The listing builds one solid part. Answer for the finished solid, in the listing's coordinates (mm). Face numbers are marked on the shaded views. A direction names the side the tool comes from. Coordinates: 2 decimals unless noted, no trailing zeros. Write each loop counter-clockwise with the first axis right and the second up, starting at its lowest first coordinate (ties: lowest second). Pieces come first, ordered by that corner, then holes. Notation, with made-up numbers: M -34,39 L -1,39 A24 ccw -1,58 Z; hole C -0.75,34 d1. An arc over 180 degrees is marked long. Put each result on its own line as item: value. Start each with the question number.
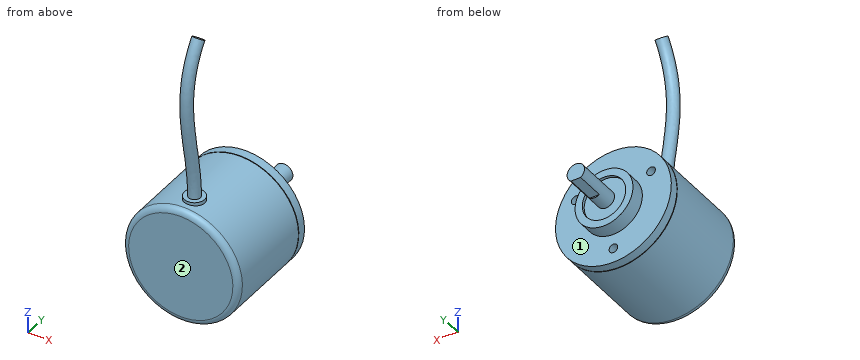
```python
from build123d import *

# Parameters (mm, degrees)
SKETCH1_R           = 20
BOSS_EXTRUDE1_DEPTH = 35
SKETCH3_R           = 10
BOSS_EXTRUDE3_DEPTH = 5
SKETCH4_R           = 7.5
CUT_EXTRUDE1_DEPTH  = 1
SKETCH5_R           = 3
BOSS_EXTRUDE4_DEPTH = 16
SKETCH6_W           = 5.83666228
SKETCH6_H           = 4.189609368
CUT_EXTRUDE2_DEPTH  = 10
SKETCH10_W          = 2.171108564
SKETCH10_H          = 0.2
SKETCH11_R          = 3.5
BOSS_EXTRUDE5_DEPTH = 21
SKETCH12_R          = 2
FILLET1_R           = 2
SKETCH24_R          = 1.5
CUT_EXTRUDE3_DEPTH  = 6


with BuildPart() as part:
    # Sketch1 → Boss-Extrude1 (new body)
    with BuildSketch(Plane(origin=(0, 0, 0), x_dir=(1, 0, 0), z_dir=(0, 1, 0))):
        with Locations(Location((0, 0, 0), (0, 0, 270))):
            Circle(SKETCH1_R)
    extrude(amount=BOSS_EXTRUDE1_DEPTH)

    # Sketch3 → Boss-Extrude3 (add)
    with BuildSketch(Plane(origin=(0, 35, 0), x_dir=(1, 0, 0), z_dir=(0, 1, 0))):
        with Locations(Location((0, 0, 0), (0, 0, 270))):
            Circle(SKETCH3_R)
    extrude(amount=BOSS_EXTRUDE3_DEPTH)

    # Sketch4 → Cut-Extrude1 (cut)
    with BuildSketch(Plane(origin=(0, 40, 0), x_dir=(1, 0, 0), z_dir=(0, 1, 0))):
        with Locations(Location((0, 0, 0), (0, 0, 270))):
            Circle(SKETCH4_R)
    extrude(amount=-CUT_EXTRUDE1_DEPTH, mode=Mode.SUBTRACT)

    # Sketch5 → Boss-Extrude4 (add)
    with BuildSketch(Plane(origin=(0, 39, 0), x_dir=(1, 0, 0), z_dir=(0, 1, 0))):
        with Locations(Location((0, 0, 0), (0, 0, 270))):
            Circle(SKETCH5_R)
    extrude(amount=BOSS_EXTRUDE4_DEPTH)

    # Sketch6 → Cut-Extrude2 (cut)
    with BuildSketch(Plane(origin=(0, 55, 0), x_dir=(1, 0, 0), z_dir=(0, 1, 0))):
        with Locations((0, 4.594804684)):
            Rectangle(SKETCH6_W, SKETCH6_H)
    extrude(amount=-CUT_EXTRUDE2_DEPTH, mode=Mode.SUBTRACT)

    # Sketch10 → Cut-Revolve1 (revolve, cut)
    with BuildSketch(Plane.XY, mode=Mode.PRIVATE) as cut_revolve1_sk:
        with Locations((20, 31.9)):
            Rectangle(SKETCH10_W, SKETCH10_H)
    revolve(cut_revolve1_sk.sketch.rotate(Axis((0, 0, 0), (0, 1, 0)), 123.557309762), axis=Axis((0, 0, 0), (0, 1, 0)), mode=Mode.SUBTRACT)

    # Sketch11 → Boss-Extrude5 (add)
    with BuildSketch(Plane.XY):
        with Locations(Location((0, 7.305759765, 0), (0, 0, 180))):
            Circle(SKETCH11_R)
    extrude(amount=BOSS_EXTRUDE5_DEPTH)

    # Sweep1: sweep along a path in Sketch13
    with BuildLine() as sweep1_path:  # in the path sketch's own coordinates; laid on its plane below (add() does not lay a ready-made edge on the line's plane)
        add(Edge.make_bspline(
            [(-21, 7.305759765), (-39.680829044, 7.305759765), (-58.658536918, -3.239081936), (-76.270922844, 9.376545434)],
            knots=[0, 0, 0, 0, 1, 1, 1, 1], degree=3))
    # Sketch12 → Sweep1 (sweep)
    with BuildSketch(Plane.XY.offset(21)):
        with Locations((0, 7.305759765)):
            Circle(SKETCH12_R)
    sweep(path=Plane(origin=(0, 0, 0), x_dir=(0, 0, -1), z_dir=(1, 0, 0)) * sweep1_path.line)

    # Fillet1
    fillet1_edges = [part.edges().sort_by_distance(p)[0] for p in [
        (0, 0, -20),
    ]]
    fillet(fillet1_edges, radius=FILLET1_R)

    # Sketch24 → Cut-Extrude3 (cut)
    with BuildSketch(Plane(origin=(0, 35, 0), x_dir=(1, 0, 0), z_dir=(0, 1, 0))):
        with Locations(Location((0, 15, 0), (0, 0, 270))):
            Circle(SKETCH24_R)
        with Locations(Location((12.990381057, -7.5, 0), (0, 0, 270))):
            Circle(SKETCH24_R)
        with Locations(Location((-12.990381057, -7.5, 0), (0, 0, 270))):
            Circle(SKETCH24_R)
    extrude(amount=-CUT_EXTRUDE3_DEPTH, mode=Mode.SUBTRACT)


solid = part.part
```
1) Given pin 1 Ø4 at (x, z) = (1.5, 30) entering from +Y; pin 2 Ø0.9 at (x, z) = (0.5, -15) entering from +Y; pin 3 Ø3.5 at (x, z) = (0, -15) entering from +Y, each flat-ended and moving along its own axis, determine where each tip first touches the part or whether it passes through.
2) For the marked faces 1 and 2, determine the directions among +Z, -Z, +X, -X, +Y, -Y from which every point of the face is accessible in a straight line to the end or side of a thin tool.
3) Straight lines are drawn through the part: probe 1 along X at (y, z) = (31, 7) (3 decimals); probe 2 along X at (y, z) = (32.7, 7.5); probe 3 along Y at (x, z) = (0.5, 10.5). For each, find the intervals that lie inside material, in ascending order.
4) A cutting plane is placed at A-A on z = 0. Write down the section's boundary in (x, y), then the cut area to 3 significant figures.
5) A cutting plane is placed at B-B on y = 41. Write down the section's boundary in (x, z).
Answers follow:
1. pin 1: stops at y = 8.83
1. pin 2: stops at y = 29
1. pin 3: stops at y = 35
2. face 1: +Y
2. face 2: +Z, -Z, +X, -X, -Y
3. probe 1: x = -18.735 to -14.405, -11.576 to 11.576, 14.405 to 18.735
3. probe 2: x = -18.54 to -14.49, -11.49 to 11.49, 14.49 to 18.54
3. probe 3: y = 0 to 35
4. outline: M -20,2 A2 ccw -18,0 L 18,0 A2 ccw 20,2 L 20,31.8 L 18.91,31.8 L 18.91,32 L 20,32 L 20,35 L 10,35 L 10,40 L 7.5,40 L 7.5,39 L 3,39 L 3,55 L -3,55 L -3,39 L -7.5,39 L -7.5,40 L -10,40 L -10,35 L -20,35 L -20,32 L -18.91,32 L -18.91,31.8 L -20,31.8 Z
4. area: 1,580 mm²
5. outline: C 0,0 d6
